```python
from build123d import *

# Parameters (mm, degrees)
SKETCH1_W           = 100
SKETCH1_H           = 100
BOSS_EXTRUDE1_DEPTH = 200
SKETCH2_R           = 25
BOSS_EXTRUDE2_DEPTH = 50
SKETCH3_R           = 3.15
BOSS_EXTRUDE3_DEPTH = 50


with BuildPart() as part:
    # Sketch1 → Boss-Extrude1 (new body)
    with BuildSketch(Plane(origin=(0, 0, 0), x_dir=(1, 0, 0), z_dir=(0, 1, 0))):
        with Locations((50, 50)):
            Rectangle(SKETCH1_W, SKETCH1_H)
    extrude(amount=BOSS_EXTRUDE1_DEPTH)

    # Sketch2 → Boss-Extrude2 (add)
    with BuildSketch(Plane.XZ):
        with Locations(Location((50, -50, 0), (0, 0, 270))):
            Circle(SKETCH2_R)
    extrude(amount=BOSS_EXTRUDE2_DEPTH)

    # Sketch3 → Boss-Extrude3 (add)
    with BuildSketch(Plane.XZ.offset(50)):
        with Locations(Location((50, -50, 0), (0, 0, 270))):
            Circle(SKETCH3_R)
    extrude(amount=BOSS_EXTRUDE3_DEPTH)


solid = part.part
```
Input: part model. Units: mm. Frame: model coordinates. A direction names the side the tool comes from. Give positions to 0.01 mm unless a question says otherwise; leave off trailing zeros. Order: outer loops, then holes, each group sorted by start corner. A loop starts at its lowest first (then second) coordinate and runs counter-clockwise, first axis right, second up. Notation, with made-up numbers: (-36, 20) -> (15, 20) arc R22 ccw to (15, 33) -> close; hole circle Ø11 at (86.5, -39.5). An arc over 180 degrees is marked (long way). Write each question's results on one line, items separated by ' | '. Start each with the question number.
Item 1: Set-up query: faces 1 (the flat face through (49, 99, -100)), 2 (the flat face through (38, 0, -73)). Return all of +Z, -Z, +X, -X, +Y, -Y with unobstructed straight access to the full face (end or side cutting, diameter ignored); none if empty.
Item 2: Cut plane B-B on z = -50. Return the cut outline in (x, y).
Item 3: Cut plane A-A on x = 50. Return the cut outline in (y, z).
Item 4: Line query: line 1 (Y direction, x = 73, z = -34); line 2 (Y direction, x = 52.5, z = -65); line 3 (X direction, y = -36.5, z = -61). Output: solid intervals per line, ascending.
Item 5: Cut plane D-D on z = -93.5. Return the cut outline in (x, y), then the cut area to 3 significant figures.
Item 6: Cut plane C-C on y = -59. Return the cut outline in (x, z), then the cut area to 3 significant figures.
Item 7: Contact query for flat-ended pins moving along their axis: P1, Ø3, axis at y = 25, z = -72, coming from the -X side; P2, Ø12, axis at x = 40.5, z = -17.5, coming from the -Y side; P3, Ø10, axis at y = -31.5, z = -61.5, coming from the -X side. Output: stop coordinate, or through.
Established:
1) face 1: -Z, +X, -X, +Y, -Y | face 2: -Y
2) outline: (0, 0) -> (25, 0) -> (25, -50) -> (46.85, -50) -> (46.85, -100) -> (53.15, -100) -> (53.15, -50) -> (75, -50) -> (75, 0) -> (100, 0) -> (100, 200) -> (0, 200) -> close
3) outline: (-100, -53.15) -> (-50, -53.15) -> (-50, -75) -> (0, -75) -> (0, -100) -> (200, -100) -> (200, 0) -> (0, 0) -> (0, -25) -> (-50, -25) -> (-50, -46.85) -> (-100, -46.85) -> close
4) line 1: 0 to 200 | line 2: -50 to 200 | line 3: 27.55 to 72.45
5) outline: (0, 0) -> (100, 0) -> (100, 200) -> (0, 200) -> close | area: 20,000 mm^2
6) outline: circle Ø6.3 at (50, -50) | area: 31.2 mm^2
7) P1: x = 0 | P2: y = 0 | P3: x = 25.86
